Build history of the part. All positions in model axes, mm. Give positions to 0.01 mm unless a question says otherwise; leave off trailing zeros. Order: outer loops, then holes, each group sorted by start corner. A loop starts at its lowest first (then second) coordinate and runs counter-clockwise, first axis right, second up. Notation, with made-up numbers: (-18, 61.25) -> (19, 61.25) arc R27 ccw to (19, 90.25) -> close; hole circle Ø1 at (-23.5, -14). An arc over 180 degrees is marked (long way). One line per item, written item: value. Start each with the question number.
(1) Saw through at B-B on x = 0. Give the cut face in (y, z).
(2) Probe line 1 (X direction, y = 0, z = 6.5); line 2 (Y direction, x = 0, z = 6.5); line 3 (X direction, y = -7.5, z = 5.5). List the from-to ranges inside material, lowest first.
(3) Saw through at A-A on y = 0. Give the cut face in (x, z).
(4) Two-plate mould, pull along X, no slides. Class faces 1 (the flat face through (30, 18, 0)), 2 (the flat face through (5.23, 21.58, 3.94)): +X half, -X half, draft (parallel to the pull), parting line (faces both ways), or undercut.
(5) Pin check, flat tips, straight feed: pin 1 (4 mm diameter, centred on y = -13.5, z = 6, fed in from +X) (3 decimals); pin 2 (2 mm diameter, centred on y = 12.5, z = 3.5, fed in from -X); pin 3 (3 mm diameter, centred on x = 59, z = 1.5, fed in from +Y). Stop position of each tip, or through.
```python
from build123d import *

# Parameters (mm, degrees)
BOSS_EXTRUDE1_DEPTH = 8
BOSS_EXTRUDE2_DEPTH = 8
CRVPATTERN1_COUNT   = 48
CRVPATTERN1_PITCH   = 5


with BuildPart() as part:
    # Sketch2 → Boss-Extrude1 (new body)
    with BuildSketch(Plane.XY):
        with BuildLine():
            Line((67.284315385, 12.320016365), (4.444661538, 23.971428489))
            ThreePointArc((4.444661538, 23.971428489), (-24.38, 0), (4.444661538, -23.971428489))
            Line((4.444661538, -23.971428489), (67.284315385, -12.320016365))
            ThreePointArc((67.284315385, -12.320016365), (77.53, 0), (67.284315385, 12.320016365))
        make_face()
        with BuildLine():
            Line((4.262353846, -22.98818696), (67.102007692, -11.336774835))
            ThreePointArc((67.102007692, -11.336774835), (76.53, 0), (67.102007692, 11.336774835))
            Line((67.102007692, 11.336774835), (4.262353846, 22.98818696))
            ThreePointArc((4.262353846, 22.98818696), (-23.38, 0), (4.262353846, -22.98818696))
        make_face(mode=Mode.SUBTRACT)
    extrude(amount=BOSS_EXTRUDE1_DEPTH)

    # Sketch4 → Boss-Extrude2 (add)
    with BuildSketch(Plane.XY):
        Polygon((4.262353846, 22.98818696), (4.360336253, 21.742033098), (6.130171006, 21.413879251), (6.668392684, 22.542071356), align=None)
    boss_extrude2 = extrude(amount=BOSS_EXTRUDE2_DEPTH)

    # CrvPattern1: Boss-Extrude2 ×48, 35 skipped
    with Locations(*[Vector(0.9832415295345763, -0.18230769209911846, 0) * (i * CRVPATTERN1_PITCH) for i in range(1, CRVPATTERN1_COUNT) if i not in (13, 14, 15, 16, 17, 18, 19, 20, 21, 22, 23, 24, 25, 26, 27, 28, 29, 30, 31, 32, 33, 34, 35, 36, 37, 38, 39, 40, 41, 42, 43, 44, 45, 46, 47)]):
        add(boss_extrude2)


solid = part.part
```
Results below:
1. outline: (-24.38, 0) -> (-23.38, 0) -> (-23.38, 8) -> (-24.38, 8) -> close; (23.38, 0) -> (24.38, 0) -> (24.38, 8) -> (23.38, 8) -> close
2. line 1: x = -24.38 to -23.38, 76.53 to 77.53
2. line 2: y = -24.38 to -23.38, 23.38 to 24.38
2. line 3: x = -23.2 to -22.14, 73.76 to 75.04
3. outline: (-24.38, 0) -> (-23.38, 0) -> (-23.38, 8) -> (-24.38, 8) -> close; (76.53, 0) -> (77.53, 0) -> (77.53, 8) -> (76.53, 8) -> close
4. face 1: draft
4. face 2: undercut
5. pin 1: stops at x = 69.975
5. pin 2: stops at x = -21.5
5. pin 3: stops at y = 14.13
